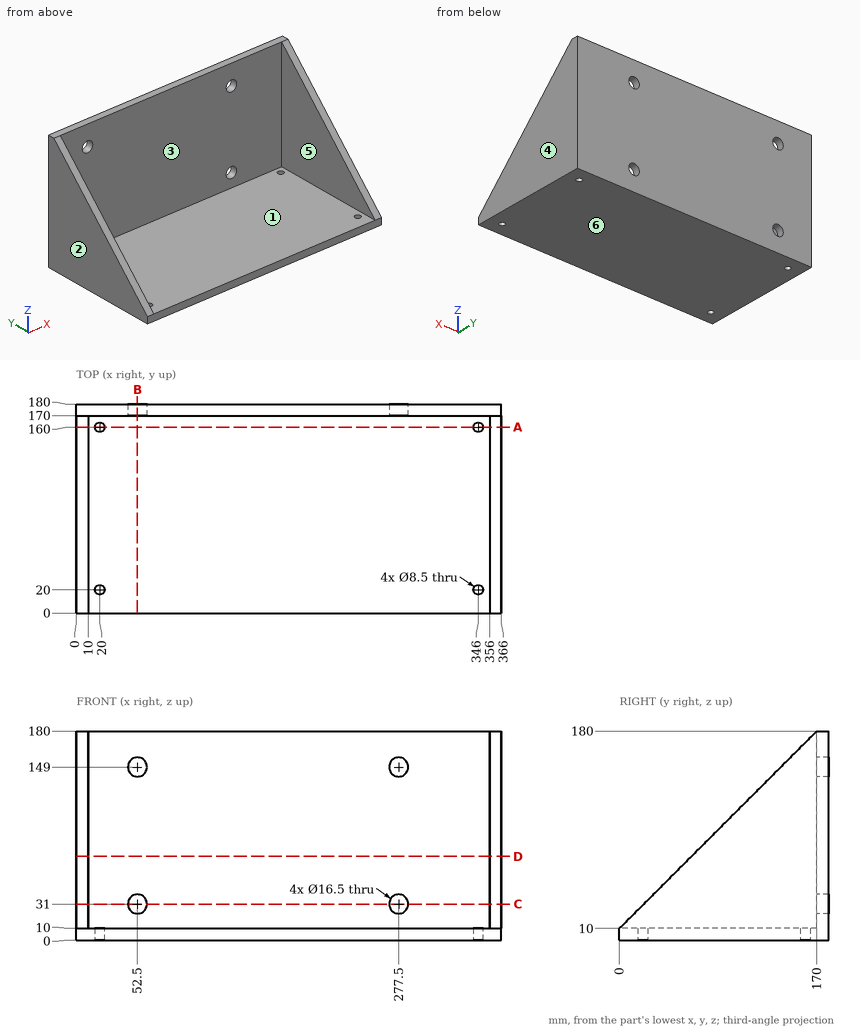
Design review of the part shown in the three views and the two pictorial views. Dimensions are in mm from the part's minimum x, y and z. A direction names the side the tool comes from. Coordinates: 2 decimals unless noted, no trailing zeros. Loops run counter-clockwise (first coordinate to the right, second up) from the corner with the lowest first, then second, coordinate; pieces in that order, holes last.
Q1. We need section A-A on y = 160. State the section outline as (x, z) points, and give its area (3 significant figures).
Reported:
outline: (0, 0) - (15.75, 0) - (15.75, 10) - (10, 10) - (10, 170) - (0, 170) - close; (24.25, 0) - (341.75, 0) - (341.75, 10) - (24.25, 10) - close; (350.25, 0) - (366, 0) - (366, 170) - (356, 170) - (356, 10) - (350.25, 10) - close
area: 6,690 mm2
Q2. The part is to be moulded in two halves that separate along X. For the marked faces 3, 4, 5 and 6, say which applies: +X half, -X half, draft (parallel to the pull), parting line (faces both ways), or undercut.
Reported:
face 3: undercut
face 4: +X half
face 5: undercut
face 6: draft
Q3. Tool access review of the marked faces 1 and 2: name each direction out of +Z, -Z, +X, -X, +Y, -Y from which nothing blocks a thin tool from reaching the whole face with its end or side.
Reported:
face 1: +Z, -Y
face 2: +Z, -Z, -X, +Y, -Y
Q4. We need section C-C on z = 31. State the section outline as (x, y) points, and give its area (3 significant figures).
Reported:
outline: (0, 21) - (10, 21) - (10, 170) - (44.25, 170) - (44.25, 180) - (0, 180) - close; (60.75, 170) - (269.25, 170) - (269.25, 180) - (60.75, 180) - close; (285.75, 170) - (356, 170) - (356, 21) - (366, 21) - (366, 180) - (285.75, 180) - close
area: 6,310 mm2
Q5. To check wall thickness, follow line 1 (Y direction, x = 346, z = 6); line 2 (Z direction, x = 277, y = 177); line 3 (X direction, y = 95, z = 52). State the ranges of each line that lie inside material, in increasing order.
Reported:
line 1: y = 0 to 15.75, 24.25 to 155.75, 164.25 to 180
line 2: z = 0 to 22.77, 39.23 to 140.77, 157.23 to 180
line 3: x = 0 to 10, 356 to 366
Q6. For pin 1 (13.5 mm diameter, centred on x = 20, y = 20, fed in from +Z); pin 2 (15 mm diameter, centred on x = 277.5, z = 31, fed in from +Y); pin 3 (5 mm diameter, centred on x = 130, z = 119.5, fed in from -Y), all flat-tipped, find the tip position at first contact; note any pin that passes through.
Reported:
pin 1: stops at z = 10
pin 2: passes through
pin 3: stops at y = 170
Q7. We need section B-B on x = 52.5. State the section outline as (y, z) points.
Reported:
outline: (0, 0) - (180, 0) - (180, 22.75) - (170, 22.75) - (170, 10) - (0, 10) - close; (170, 39.25) - (180, 39.25) - (180, 140.75) - (170, 140.75) - close; (170, 157.25) - (180, 157.25) - (180, 180) - (170, 180) - close
Q8. We need section D-D on z = 72. State the section outline as (x, y) points, and give its area (3 significant figures).
Reported:
outline: (0, 62) - (10, 62) - (10, 170) - (356, 170) - (356, 62) - (366, 62) - (366, 180) - (0, 180) - close
area: 5,820 mm2
